Geometry: final body of the model. Coordinates: model frame, mm. A direction names the side the tool comes from. Give positions to 0.01 mm unless a question says otherwise; leave off trailing zeros. Write each loop counter-clockwise with the first axis right and the second up, starting at its lowest first coordinate (ties: lowest second). Pieces come first, ordered by that corner, then holes. Notation, with made-up numbers: (83.25, 20.25) -> (117.25, 20.25) arc R20 ccw to (117.25, 24.25) -> close; hole circle Ø7 at (-29, -9.5). An arc over 180 degrees is marked (long way). Answer as a JSON object with one key per item and string values. Group by question number.
(1) Section query C-C on x = -4. Output: boundary loops of the cut face in (y, z), plus the area to 3 significant figures.
(2) Contact query for flat-ended pins moving along their axis: pin 1 Ø8 at (x, z) = (-1.5, 13) entering from +Y; pin 2 Ø3 at (x, y) = (-6, 0.5) entering from +Z; pin 3 Ø2 at (y, z) = (-0.5, 12) entering from +X. Output: stop coordinate, or through.
(3) Draft query along X for faces 4 (the face through (0, 0, 10)), 5 (the face through (4, 4, 15)), 6 (the face through (-8, 0, 5)). Return one class per face: +X half, -X half, draft (parallel to the pull), parting line (faces both ways), or undercut.
(4) Material intervals for probe 1 along Y at (x, z) = (0, 3); probe 2 along Y at (x, z) = (2.75, 6.25); probe 3 along X at (y, z) = (-3.75, 3), sorted ascending.
(5) Section query D-D on x = 2.25. Output: boundary loops of the cut face in (y, z).
(6) Section query A-A on z = 3.5. Output: boundary loops of the cut face in (x, y).
(7) Section query B-B on y = 4. Output: boundary loops of the cut face in (x, z).
(8) Set-up query: faces 1 (the face through (0, 0, 9)), 2 (the face through (-5.6, -5.2, 12.5)), 3 (the face through (-4, 4, 15)). Return all of +Z, -Z, +X, -X, +Y, -Y with unobstructed straight access to the full face (end or side cutting, diameter ignored); none if empty.
from build123d import *

# Parameters (mm, degrees)
SKETCH1_W           = 16
SKETCH1_H           = 16
BOSS_EXTRUDE1_DEPTH = 10
SKETCH2_R           = 2
BOSS_EXTRUDE3_DEPTH = 5
SKETCH3_W           = 13.5
SKETCH3_H           = 13.650151982
CUT_EXTRUDE1_DEPTH  = 9
SKETCH4_R           = 3.7
SKETCH4_R_2         = 2.7
BOSS_EXTRUDE4_DEPTH = 9


with BuildPart() as part:
    # Sketch1 → Boss-Extrude1 (new body)
    with BuildSketch(Plane.XY):
        Rectangle(SKETCH1_W, SKETCH1_H)
    extrude(amount=BOSS_EXTRUDE1_DEPTH)

    # Sketch2 → Boss-Extrude3 (add)
    with BuildSketch(Plane.XY.offset(10)):
        with Locations((-4, 4)):
            Circle(SKETCH2_R)
        with Locations((4, 4)):
            Circle(SKETCH2_R)
        with Locations((4, -4)):
            Circle(SKETCH2_R)
        with Locations((-4, -4)):
            Circle(SKETCH2_R)
    extrude(amount=BOSS_EXTRUDE3_DEPTH)

    # Sketch3 → Cut-Extrude1 (cut)
    with BuildSketch(Plane(origin=(0, 0, 0), x_dir=(-1, 0, 0), z_dir=(0, 0, -1))):
        Rectangle(SKETCH3_W, SKETCH3_H)
    extrude(amount=-CUT_EXTRUDE1_DEPTH, mode=Mode.SUBTRACT)

    # Sketch4 → Boss-Extrude4 (add)
    with BuildSketch(Plane(origin=(0, 0, 9), x_dir=(-1, 0, 0), z_dir=(0, 0, -1))):
        with Locations(Location((0, 0, 0), (0, 0, 180))):
            Circle(SKETCH4_R)
        Circle(SKETCH4_R_2, mode=Mode.SUBTRACT)
    extrude(amount=BOSS_EXTRUDE4_DEPTH)


solid = part.part
Answer list:
{
 "1": {"outline": "(-8, 0) -> (-6.83, 0) -> (-6.83, 9) -> (6.83, 9) -> (6.83, 0) -> (8, 0) -> (8, 10) -> (6, 10) -> (6, 15) -> (2, 15) -> (2, 10) -> (-2, 10) -> (-2, 15) -> (-6, 15) -> (-6, 10) -> (-8, 10) -> close", "area": "77.1 mm2"},
 "2": {"pin 1": "y = 8", "pin 2": "z = 10", "pin 3": "through"},
 "3": {"face 4": "undercut", "face 5": "draft", "face 6": "-X half"},
 "4": {"probe 1": "-8 to -6.83, -3.7 to -2.7, 2.7 to 3.7, 6.83 to 8", "probe 2": "-8 to -6.83, -2.48 to 2.48, 6.83 to 8", "probe 3": "-8 to -6.75, 6.75 to 8"},
 "5": {"outline": "(-8, 0) -> (-6.83, 0) -> (-6.83, 9) -> (-2.94, 9) -> (-2.94, 0) -> (-1.49, 0) -> (-1.49, 9) -> (1.49, 9) -> (1.49, 0) -> (2.94, 0) -> (2.94, 9) -> (6.83, 9) -> (6.83, 0) -> (8, 0) -> (8, 10) -> (4.97, 10) -> (4.97, 15) -> (3.03, 15) -> (3.03, 10) -> (-3.03, 10) -> (-3.03, 15) -> (-4.97, 15) -> (-4.97, 10) -> (-8, 10) -> close"},
 "6": {"outline": "(-8, -8) -> (8, -8) -> (8, 8) -> (-8, 8) -> close; circle Ø7.4 at (0, 0); hole (-6.75, -6.83) -> (6.75, -6.83) -> (6.75, 6.83) -> (-6.75, 6.83) -> close; hole circle Ø5.4 at (0, 0)"},
 "7": {"outline": "(-8, 0) -> (-6.75, 0) -> (-6.75, 9) -> (6.75, 9) -> (6.75, 0) -> (8, 0) -> (8, 10) -> (6, 10) -> (6, 15) -> (2, 15) -> (2, 10) -> (-2, 10) -> (-2, 15) -> (-6, 15) -> (-6, 10) -> (-8, 10) -> close"},
 "8": {"face 1": "-Z", "face 2": "+Z", "face 3": "+Z, +X, -X, +Y, -Y"}
}
